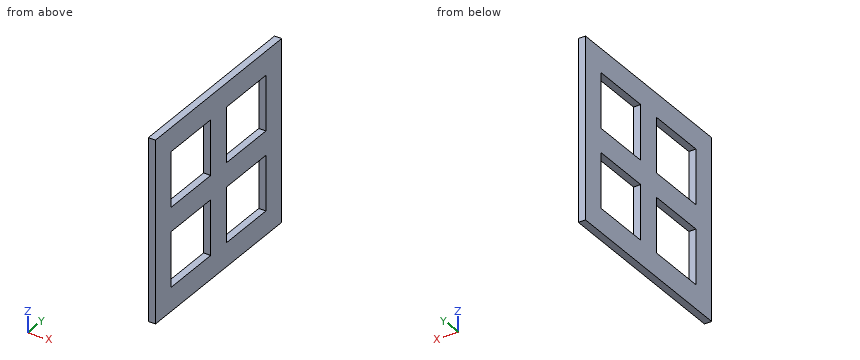
from build123d import *

# Parameters (mm, degrees)
F0_W     = 8
F0_H     = 7.633
F1_DEPTH = 0.3


with BuildPart() as f1:
    # F0 (on Right) → F1 (new body)
    with BuildSketch(Plane.YZ):
        with Locations((-11.22477, -15.256895)):
            Rectangle(F0_W, F0_H)
        Polygon((-14.22477, -14.751895), (-14.22477, -12.440395), (-11.72477, -12.440395), (-10.72477, -12.440395), (-8.22477, -12.440395), (-8.22477, -14.751895), (-8.22477, -15.761895), (-8.22477, -18.073395), (-10.72477, -18.073395), (-11.72477, -18.073395), (-14.22477, -18.073395), (-14.22477, -15.761895), align=None, mode=Mode.SUBTRACT)
        Polygon((-10.72477, -12.440395), (-11.72477, -12.440395), (-11.72477, -14.751895), (-14.22477, -14.751895), (-14.22477, -15.761895), (-11.72477, -15.761895), (-11.72477, -18.073395), (-10.72477, -18.073395), (-10.72477, -15.761895), (-8.22477, -15.761895), (-8.22477, -14.751895), (-10.72477, -14.751895), align=None)
    extrude(amount=F1_DEPTH)


solid = f1.part
Here's how the part is built. I have some questions about the finished solid (model axes, mm). Coordinates: 2 decimals unless noted, no trailing zeros. Loops run counter-clockwise (first coordinate to the right, second up) from the corner with the lowest first, then second, coordinate; pieces in that order, holes last. Notation, with made-up numbers: (20, 54) -> (63, 54) arc R12 cw to (63, 64) -> close; hole circle Ø6 at (-38, -14.75). An arc over 180 degrees is marked (long way). Use one line per item in the form item = value. Start each with the question number.
(1) If we section it at B-B (x = 0.15): Please give me the cut outline in (y, z), then the cut area to 3 significant figures.
(2) If we section it at A-A (z = -17.25): Please give me the cut outline in (x, y).
(3) Please list where these lines run through material, in increasing order: line 1 along Y through (x, z) = (0.2, -13.75); line 2 along Z through (x, y) = (0.1, -10.5).
(4) If we section it at C-C (y = -12.5): Please give me the cut outline in (x, z), then the cut area to 3 significant figures.
Verdict:
q1.outline = (-15.22, -19.07) -> (-7.22, -19.07) -> (-7.22, -11.44) -> (-15.22, -11.44) -> close; hole (-14.22, -18.07) -> (-11.72, -18.07) -> (-11.72, -15.76) -> (-14.22, -15.76) -> close; hole (-14.22, -14.75) -> (-11.72, -14.75) -> (-11.72, -12.44) -> (-14.22, -12.44) -> close; hole (-10.72, -18.07) -> (-8.22, -18.07) -> (-8.22, -15.76) -> (-10.72, -15.76) -> close; hole (-10.72, -14.75) -> (-8.22, -14.75) -> (-8.22, -12.44) -> (-10.72, -12.44) -> close
q1.area = 37.9 mm²
q2.outline = (0, -15.22) -> (0.3, -15.22) -> (0.3, -14.22) -> (0, -14.22) -> close; (0, -11.72) -> (0.3, -11.72) -> (0.3, -10.72) -> (0, -10.72) -> close; (0, -8.22) -> (0.3, -8.22) -> (0.3, -7.22) -> (0, -7.22) -> close
q3.line_1 = -15.22 to -14.22, -11.72 to -10.72, -8.22 to -7.22
q3.line_2 = -19.07 to -18.07, -15.76 to -14.75, -12.44 to -11.44
q4.outline = (0, -19.07) -> (0.3, -19.07) -> (0.3, -18.07) -> (0, -18.07) -> close; (0, -15.76) -> (0.3, -15.76) -> (0.3, -14.75) -> (0, -14.75) -> close; (0, -12.44) -> (0.3, -12.44) -> (0.3, -11.44) -> (0, -11.44) -> close
q4.area = 0.903 mm²
